```python
from build123d import *

# Parameters (mm, degrees)
F0_W     = 63.325
F0_H     = 90.31
F0_W_2   = 50.625042
F0_H_2   = 51.194
F1_DEPTH = 0.82


with BuildPart() as f1:
    # F0 (on Front) → F1 (new body)
    with BuildSketch(Plane.XZ):
        with Locations((31.6625, 45.155)):
            Rectangle(F0_W, F0_H)
        with Locations((31.662521, 31.947)):
            Rectangle(F0_W_2, F0_H_2, mode=Mode.SUBTRACT)
        Polygon((6.34999, 63.894056), (6.349968, 77.610057), (56.97501, 77.610057), (56.975032, 63.894056), align=None, mode=Mode.SUBTRACT)
    extrude(amount=F1_DEPTH)


solid = f1.part
```
Verification items for the finished model (mm, model axes). Give positions to 0.01 mm unless a question says otherwise; leave off trailing zeros. Loops run counter-clockwise (first coordinate to the right, second up) from the corner with the lowest first, then second, coordinate; pieces in that order, holes last.
1. Thickness scan on line 1 (Z direction, x = 15, y = -0.4); line 2 (X direction, y = -0.6, z = 31) (3 decimals). Record the ranges inside material, lowest first.
2. Section check C-C, the plane y = -0.15. Enter the section's corners in (x, z) (3 decimals).
3. Section check B-B, the plane z = 17. Enter the section's corners in (x, y) (3 decimals), then the cut area to 3 significant figures.
4. Section check A-A, the plane x = 41.5. Enter the section's corners in (y, z).
Geometry says:
1. line 1: z = 0 to 6.35, 57.54 to 63.89, 77.61 to 90.31
1. line 2: x = 0 to 6.35, 56.975 to 63.325
2. outline: (0, 0) - (63.325, 0) - (63.325, 90.31) - (0, 90.31) - close; hole (6.35, 6.35) - (56.975, 6.35) - (56.975, 57.544) - (6.35, 57.544) - close; hole (6.35, 63.894) - (56.975, 63.894) - (56.975, 77.61) - (6.35, 77.61) - close
3. outline: (0, -0.82) - (6.35, -0.82) - (6.35, 0) - (0, 0) - close; (56.975, -0.82) - (63.325, -0.82) - (63.325, 0) - (56.975, 0) - close
3. area: 10.4 mm2
4. outline: (-0.82, 0) - (0, 0) - (0, 6.35) - (-0.82, 6.35) - close; (-0.82, 57.54) - (0, 57.54) - (0, 63.89) - (-0.82, 63.89) - close; (-0.82, 77.61) - (0, 77.61) - (0, 90.31) - (-0.82, 90.31) - close
